Verification items for the finished model (mm, model axes). Face numbers are marked on the shaded views. A direction names the side the tool comes from. Give positions to 0.01 mm unless a question says otherwise; leave off trailing zeros. Write each loop counter-clockwise with the first axis right and the second up, starting at its lowest first coordinate (ties: lowest second). Pieces come first, ordered by that corner, then holes. Notation, with made-up numbers: M 60,44 L 111,44 A25 ccw 111,61 Z; hole C 83,83.25 d7. An arc over 180 degrees is marked long. Write item = value, one per line.
from build123d import *

# Parameters (mm, degrees)
CROQUIS1_W                 = 15
CROQUIS1_H                 = 43
SALIENTE_EXTRUIR1_DEPTH    = 12
CROQUIS2_W                 = 15
CROQUIS2_H                 = 4
SALIENTE_EXTRUIR2_DEPTH    = 33
CROQUIS3_R                 = 1.5
CORTAR_EXTRUIR1_DEPTH      = 13
CORTAR_EXTRUIR2_DEPTH      = 3.5
REDONDEO1_R                = 3
CORTAR_EXTRUIR3_DEPTH      = 63.691705991
CORTAR_EXTRUIR3_DEPTH_BACK = 63.691705991
CROQUIS5_R                 = 1.5


with BuildPart() as part:
    # Croquis1 → Saliente-Extruir1 (new body)
    with BuildSketch(Plane(origin=(0, 0, 0), x_dir=(1, 0, 0), z_dir=(0, 1, 0))):
        Rectangle(CROQUIS1_W, CROQUIS1_H)
    extrude(amount=SALIENTE_EXTRUIR1_DEPTH)

    # Croquis2 → Saliente-Extruir2 (add)
    with BuildSketch(Plane(origin=(0, 12, 0), x_dir=(1, 0, 0), z_dir=(0, 1, 0))):
        with Locations((0, 19.5)):
            Rectangle(CROQUIS2_W, CROQUIS2_H)
        with Locations((0, -19.5)):
            Rectangle(CROQUIS2_W, CROQUIS2_H)
    extrude(amount=SALIENTE_EXTRUIR2_DEPTH)

    # Croquis3 → Cortar-Extruir1 (cut)
    with BuildSketch(Plane.XZ):
        with Locations(Location((0, 14.5, 0), (0, 0, 270))):
            Circle(CROQUIS3_R)
        with Locations(Location((0, -14.5, 0), (0, 0, 270))):
            Circle(CROQUIS3_R)
    extrude(amount=-CORTAR_EXTRUIR1_DEPTH, mode=Mode.SUBTRACT)

    # Croquis4 → Cortar-Extruir2 (cut)
    with BuildSketch(Plane(origin=(0, 12, 0), x_dir=(1, 0, 0), z_dir=(0, 1, 0))):
        Polygon((3.464101615, 14.5), (1.732050808, 17.5), (-1.732050808, 17.5), (-3.464101615, 14.5), (-1.732050808, 11.5), (1.732050808, 11.5), align=None)
        Polygon((3.464101615, -14.5), (1.732050808, -11.5), (-1.732050808, -11.5), (-3.464101615, -14.5), (-1.732050808, -17.5), (1.732050808, -17.5), align=None)
    extrude(amount=-CORTAR_EXTRUIR2_DEPTH, mode=Mode.SUBTRACT)

    # Redondeo1
    redondeo1_edges = [part.edges().sort_by_distance(p)[0] for p in [
        (-7.5, 22.5, -21.5),
        (7.5, 22.5, -21.5),
        (7.5, 22.5, 21.5),
        (-7.5, 22.5, 21.5),
    ]]
    fillet(redondeo1_edges, radius=REDONDEO1_R)

    # Croquis5 → Cortar-Extruir3 (cut, two sides: drawn at the far end of the back side and taken through both)
    with BuildSketch(Plane(origin=(0, 0, -21.5), x_dir=(-1, 0, 0), z_dir=(0, 0, -1)).offset(-CORTAR_EXTRUIR3_DEPTH_BACK)):
        with Locations((0, 41.5)):
            Circle(CROQUIS5_R)
    extrude(amount=CORTAR_EXTRUIR3_DEPTH + CORTAR_EXTRUIR3_DEPTH_BACK, mode=Mode.SUBTRACT)


solid = part.part
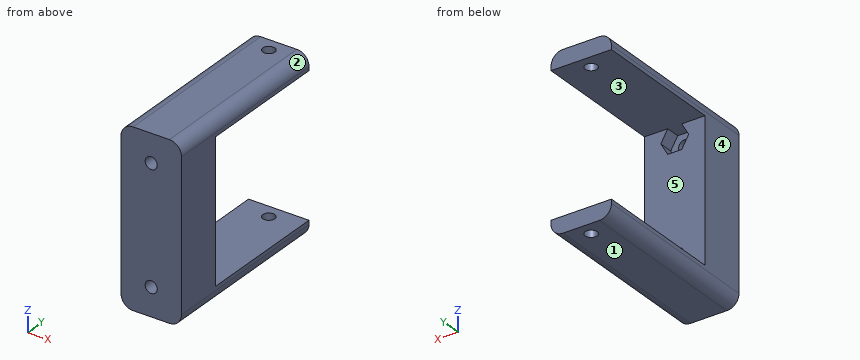
1) Cross-section at C-C on y = 41.5. Record the boundary of the cut face in (x, z).
From the geometry:
outline = M -7.5,-18.5 A3 ccw -4.5,-21.5 L -1.5,-21.5 L -1.5,-17.5 L -7.5,-17.5 Z; M -7.5,17.5 L -1.5,17.5 L -1.5,21.5 L -4.5,21.5 A3 ccw -7.5,18.5 Z; M 1.5,-21.5 L 4.5,-21.5 A3 ccw 7.5,-18.5 L 7.5,-17.5 L 1.5,-17.5 Z; M 1.5,17.5 L 7.5,17.5 L 7.5,18.5 A3 ccw 4.5,21.5 L 1.5,21.5 Z
2) Cross-section at B-B on x = 0. Record the boundary of the cut face in (y, z).
From the geometry:
outline = M 0,-21.5 L 40,-21.5 L 40,-17.5 L 8.5,-17.5 L 8.5,-16 L 0,-16 Z; M 0,-13 L 8.5,-13 L 8.5,-11.5 L 12,-11.5 L 12,11.5 L 8.5,11.5 L 8.5,13 L 0,13 Z; M 0,16 L 8.5,16 L 8.5,17.5 L 40,17.5 L 40,21.5 L 0,21.5 Z; M 43,-21.5 L 45,-21.5 L 45,-17.5 L 43,-17.5 Z; M 43,17.5 L 45,17.5 L 45,21.5 L 43,21.5 Z
3) Depth check by flat-ended pin: P1, Ø6.5, axis at x = 1.5, z = -14, coming from the +Y side; P2, Ø2.5, axis at x = 0, z = -14.5, coming from the -Y side; P3, Ø1.8, axis at x = 1, z = 14, coming from the +Y side. Enter the tip coordinate at first touch or a pass-through.
From the geometry:
P1 = 12
P2 = through
P3 = 8.5
4) Draft check along Z on the marked faces 1, 2 and 3. Enter one of: +Z half, -Z half, draft (parallel to the pull), parting line (faces both ways), or undercut.
From the geometry:
face_1 = -Z half
face_2 = +Z half
face_3 = undercut
5) Cross-section at D-D on y = 10. Record the boundary of the cut face in (x, z), plus the area to 3 significant figures.
From the geometry:
outline = M -7.5,-18.5 A3 ccw -4.5,-21.5 L 4.5,-21.5 A3 ccw 7.5,-18.5 L 7.5,18.5 A3 ccw 4.5,21.5 L -4.5,21.5 A3 ccw -7.5,18.5 Z; hole M -3.46,-14.5 L -1.73,-17.5 L 1.73,-17.5 L 3.46,-14.5 L 1.73,-11.5 L -1.73,-11.5 Z; hole M -3.46,14.5 L -1.73,11.5 L 1.73,11.5 L 3.46,14.5 L 1.73,17.5 L -1.73,17.5 Z
area = 575 mm^2
6) Tool access check on the marked faces 4 and 5. Record the directions out of +Z, -Z, +X, -X, +Y, -Y that give a thin tool (end or side, any length) a straight path to the whole face; none if there is none.
From the geometry:
face_4 = +Z, -Z, -X, +Y, -Y
face_5 = +X, -X, +Y
7) Material ranges on probe 1 along X at (y, z) = (4.75, -14.5); probe 2 along Z at (x, y) = (0.5, 33); probe 3 along Y at (x, z) = (0, 18.9), recorded low to high. Write a range as from..to.
From the geometry:
probe_1 = -7.5..-1.5, 1.5..7.5
probe_2 = -21.5..-17.5, 17.5..21.5
probe_3 = 0..40, 43..45
8) Cross-section at A-A on y = 30. Record the boundary of the cut face in (x, z).
From the geometry:
outline = M -7.5,-18.5 A3 ccw -4.5,-21.5 L 4.5,-21.5 A3 ccw 7.5,-18.5 L 7.5,-17.5 L -7.5,-17.5 Z; M -7.5,17.5 L 7.5,17.5 L 7.5,18.5 A3 ccw 4.5,21.5 L -4.5,21.5 A3 ccw -7.5,18.5 Z
